Read the model definition and answer for the solid it produces. Units are mm, in the model's axes. A direction names the side the tool comes from. Coordinates: 2 decimals unless noted, no trailing zeros. Loops run counter-clockwise (first coordinate to the right, second up) from the corner with the lowest first, then second, coordinate; pieces in that order, holes last. Notation, with made-up numbers: (43.25, -32.5) - (92.25, -32.5) arc R15 cw to (92.25, -10.5) - close; hole circle Ø8 at (85, -16). An arc over 180 degrees is marked (long way). Use one line per item in the form item = value. Start each with the question number.
1) A cutting plane is placed at C-C (y = 0). Give the vertices of the cut face in (x, z), and give its area (3 significant figures).
2) Each of these flat-tipped pins is pushed along its axis until it touches: P1, Ø2, axis at y = 5, z = 1.5, coming from the +X side; P2, Ø1.5, axis at x = 1, z = 0.5, coming from the +Y side; P3, Ø8, axis at x = 1, y = 6.5, coming from the +Z side. Where does it stop, or does it pass through?
3) Which of the six approach directions +Z, -Z, +X, -X, +Y, -Y give full straight-line access (tool end or side, diameter ignored) to faces 4 (the face through (0, 13.95, 1)), 5 (the face through (0, 9, 3.6)), 6 (the face through (0, 8, 2))?
4) The mould has two halves that part along X. Classify faces 1 (the face through (0, -16.95, 4)), 2 (the face through (16.75, 0, 4)), 3 (the face through (0, -13.95, 5)): released by +X, released by -X, zero draft, split by the parting line, or undercut.
5) Consider line 1 (X direction, y = -2.5, z = 1.8); line 2 (X direction, y = 7.5, z = 4.7); line 3 (Y direction, x = 6.5, z = 2.3). Determine where each line is inside the solid, lowest interval first.
6) A cutting plane is placed at B-B (z = 4.2). Give the vertices of the cut face in (x, y), and give its area (3 significant figures).
7) A cutting plane is placed at A-A (x = 13). Give the vertices of the cut face in (y, z), and give its area (3 significant figures).
8) A cutting plane is placed at D-D (y = 11). Give the vertices of the cut face in (x, z), and give its area (3 significant figures).
Autodesk Fusion 360 part; units mm, degrees
sketch "Esquisse1" plane through (0, 0, 0) normal (0, 0, 1) x (1, 0, 0)
  line L0 (13.5, 8) -> (-13.5, 8)
  line L1 (-13.5, 8) -> (-13.5, -8)
  line L2 (-13.5, -8) -> (13.5, -8)
  line L3 (13.5, -8) -> (13.5, 8)
  line L4 (13.5, 8) -> (-13.5, -8) construction
  line L5 (-13.5, 8) -> (13.5, -8) construction
  line L6 (13.75, 13.95) -> (-13.75, 13.95)
  line L7 (-13.75, 13.95) -> (-13.75, -13.95)
  line L8 (-13.75, -13.95) -> (13.75, -13.95)
  line L9 (13.75, -13.95) -> (13.75, 13.95)
  line L10 (13.75, 13.95) -> (-13.75, -13.95) construction
  line L11 (-13.75, 13.95) -> (13.75, -13.95) construction
  line L12 (-16.75, -16.95) -> (16.75, -16.95)
  line L13 (16.75, -16.95) -> (16.75, 16.95)
  line L14 (16.75, 16.95) -> (-16.75, 16.95)
  line L15 (-16.75, 16.95) -> (-16.75, -16.95)
  dimension "d1" = 27
  dimension "d2" = 16
  dimension "d3" = 27.5
  dimension "d4" = 27.9
  dimension "d5" = 3
extrude "Extrusion1" add sketch "Esquisse1" along normal blind 3.6 contours L6 L7 L8 L9
extrude "Extrusion2" add sketch "Esquisse1" along normal blind 5.6 contours L12 L13 L14 L15
extrude "Extrusion3" cut sketch "Esquisse1" along normal blind 2.6 contours L12 L13 L14 L15
equation "d6 = 2.6 mm + 1 mm"
equation "d8 = 2.6 mm + 3 mm"
Found:
q1.outline = (-16.75, 2.6) - (-13.75, 2.6) - (-13.75, 0) - (-13.5, 0) - (-13.5, 3.6) - (-13.75, 3.6) - (-13.75, 5.6) - (-16.75, 5.6) - close; (13.5, 0) - (13.75, 0) - (13.75, 2.6) - (16.75, 2.6) - (16.75, 5.6) - (13.75, 5.6) - (13.75, 3.6) - (13.5, 3.6) - close
q1.area = 19.8 mm^2
q2.P1 = 13.75
q2.P2 = 13.95
q2.P3 = 3.6
q3.face_4 = -Z, +X, -X, +Y
q3.face_5 = +Z
q3.face_6 = +Z, -Z
q4.face_1 = zero draft
q4.face_2 = released by +X
q4.face_3 = undercut
q5.line_1 = -13.75 to -13.5, 13.5 to 13.75
q5.line_2 = -16.75 to -13.75, 13.75 to 16.75
q5.line_3 = -13.95 to -8, 8 to 13.95
q6.outline = (-16.75, -16.95) - (16.75, -16.95) - (16.75, 16.95) - (-16.75, 16.95) - close; hole (-13.75, -13.95) - (13.75, -13.95) - (13.75, 13.95) - (-13.75, 13.95) - close
q6.area = 368 mm^2
q7.outline = (-16.95, 2.6) - (-13.95, 2.6) - (-13.95, 0) - (-8, 0) - (-8, 3.6) - (-13.95, 3.6) - (-13.95, 5.6) - (-16.95, 5.6) - close; (8, 0) - (13.95, 0) - (13.95, 2.6) - (16.95, 2.6) - (16.95, 5.6) - (13.95, 5.6) - (13.95, 3.6) - (8, 3.6) - close
q7.area = 60.8 mm^2
q8.outline = (-16.75, 2.6) - (-13.75, 2.6) - (-13.75, 0) - (13.75, 0) - (13.75, 2.6) - (16.75, 2.6) - (16.75, 5.6) - (13.75, 5.6) - (13.75, 3.6) - (-13.75, 3.6) - (-13.75, 5.6) - (-16.75, 5.6) - close
q8.area = 117 mm^2
